Source: CAD feature listing. Evaluate the final solid. Frame: model axes, mm. Face numbers are marked on the shaded views. A direction names the side the tool comes from. Give positions to 0.01 mm unless a question says otherwise; leave off trailing zeros. Write each loop counter-clockwise with the first axis right and the second up, starting at its lowest first coordinate (ties: lowest second). Pieces come first, ordered by that corner, then holes.
```python
from build123d import *

# Parameters (mm, degrees)
SKETCH1_R                 = 7.5
EXTRUDE1_DEPTH            = 3
SKETCH2_R                 = 30
EXTRUDE2_DEPTH            = 6
SKETCH3_R                 = 18.5
CUT_EXTRUDE1_DEPTH        = 45.09081537
CUT_EXTRUDE2_DEPTH        = 45.09081537
SKETCH8_R                 = 18.75
EXTRUDE3_DEPTH            = 45.09081537
CIRPATTERN1_COUNT         = 5
SKETCH5_R                 = 3.05
CUT_EXTRUDE3_DEPTH        = 44.640169222
M3X0_5_TAPPED_HOLE1_D     = 2.5
M3X0_5_TAPPED_HOLE1_DEPTH = 7.5
M3X0_5_TAPPED_HOLE1_TIP   = 0.751075774


with BuildPart() as part:
    # Sketch1 → Extrude1 (new, symmetric)
    with BuildSketch(Plane.XY):
        Circle(SKETCH1_R)
    extrude(amount=EXTRUDE1_DEPTH, both=True)

    # Sketch2 → Extrude2 (add)
    with BuildSketch(Plane(origin=(0, 0, -3), x_dir=(-1, 0, 0), z_dir=(0, 0, -1))):
        Circle(SKETCH2_R)
    extrude(amount=EXTRUDE2_DEPTH)

    # Sketch3 → Cut-Extrude1 (cut, through all)
    with BuildSketch(Plane(origin=(0, 0, -9), x_dir=(-1, 0, 0), z_dir=(0, 0, -1))):
        with Locations((0, -38)):
            Circle(SKETCH3_R)
    cut_extrude1 = extrude(amount=-CUT_EXTRUDE1_DEPTH, mode=Mode.SUBTRACT)

    # Sketch4 → Cut-Extrude2 (cut, through all)
    with BuildSketch(Plane(origin=(0, 0, -9), x_dir=(-1, 0, 0), z_dir=(0, 0, -1))):
        with BuildLine():
            Line((6.794236298, -13.604718046), (15.549680784, -25.655553542))
            ThreePointArc((15.549680784, -25.655553542), (17.633557569, -24.270509831), (19.594765756, -22.71662728))
            Line((19.594765756, -22.71662728), (10.83932127, -10.665791785))
            ThreePointArc((10.83932127, -10.665791785), (7.347315654, -10.11271243), (6.794236298, -13.604718046))
        make_face()
    cut_extrude2 = extrude(amount=-CUT_EXTRUDE2_DEPTH, mode=Mode.SUBTRACT)

    # Sketch8 → Extrude3 (cut, through all)
    with BuildSketch(Plane(origin=(0, 0, -9), x_dir=(-1, 0, 0), z_dir=(0, 0, -1))):
        with Locations((0, -38)):
            Circle(SKETCH8_R)
    extrude3 = extrude(amount=-EXTRUDE3_DEPTH, mode=Mode.SUBTRACT)

    # CirPattern1: Cut-Extrude1, Cut-Extrude2, Extrude3 ×5 about axis
    cirpattern1_axis = Axis((0, 0, 0), (0, 0, 1))
    add([cut_extrude1.rotate(cirpattern1_axis, i * 360 / CIRPATTERN1_COUNT) for i in range(1, CIRPATTERN1_COUNT)], mode=Mode.SUBTRACT)
    add([cut_extrude2.rotate(cirpattern1_axis, i * 360 / CIRPATTERN1_COUNT) for i in range(1, CIRPATTERN1_COUNT)], mode=Mode.SUBTRACT)
    add([extrude3.rotate(cirpattern1_axis, i * 360 / CIRPATTERN1_COUNT) for i in range(1, CIRPATTERN1_COUNT)], mode=Mode.SUBTRACT)

    # Sketch5 → Cut-Extrude3 (cut, through all)
    with BuildSketch(Plane(origin=(0, 0, -9), x_dir=(-1, 0, 0), z_dir=(0, 0, -1))):
        Circle(SKETCH5_R)
    extrude(amount=-CUT_EXTRUDE3_DEPTH, mode=Mode.SUBTRACT)

    # M3x0.5 Tapped Hole1
    with Locations(Plane(origin=(0, 7.5, 0), x_dir=(-1, 0, 0), z_dir=(0, 1, 0))):
        with Locations((0, 0)):
            Hole(M3X0_5_TAPPED_HOLE1_D / 2, depth=M3X0_5_TAPPED_HOLE1_DEPTH)
            with Locations((0, 0, -(M3X0_5_TAPPED_HOLE1_DEPTH + M3X0_5_TAPPED_HOLE1_TIP / 2))):  # 118° drill point
                Cone(0, M3X0_5_TAPPED_HOLE1_D / 2, M3X0_5_TAPPED_HOLE1_TIP, mode=Mode.SUBTRACT)


solid = part.part
```
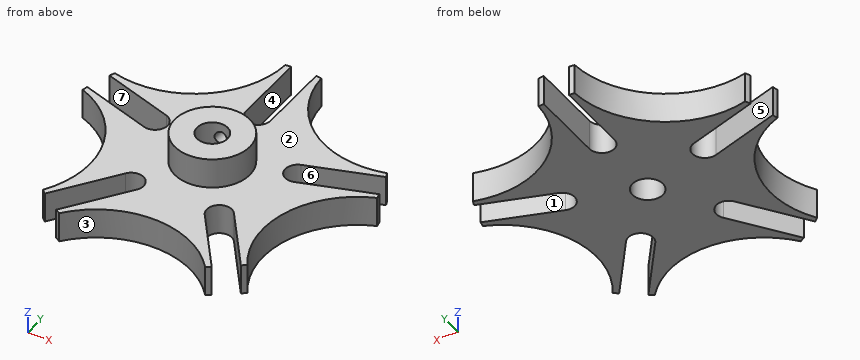
1. Mould query, pull axis Y, two halves, no side actions, for the marked faces 1, 2 and 3. Classes: +Y half, -Y half, draft (parallel to the pull), parting line (faces both ways), or undercut.
2. Line query: L1, parallel to Z at x = 0, y = 6.55; L2, parallel to X at y = 0.5, z = 2; L3, parallel to Y at x = 0, z = -2. Output: solid intervals per line, ascending.
3. Contact query for flat-ended pins moving along their axis: P1, Ø12, axis at x = 14.5, y = 11.5, coming from the +Z side; P2, Ø6, axis at x = 6, z = 1, coming from the -Y side; P3, Ø2, axis at x = 0, z = 0, coming from the -Y side; P4, Ø2, axis at x = 17, z = -0.5, coming from the -Y side. Output: stop coordinate, or through.
4. Cut plane D-D, the plane y = -16.5. Return the cut outline in (x, z), then the cut area to 3 significant figures.
5. Cut plane B-B, the plane y = 0. Return the cut outline in (x, z).
6. Access query for the marked faces 4, 5, 6 and 7. Directions: +Z, -Z, +X, -X, +Y, -Y. A direction counts if a zero-diameter tool reaches every point of the face in a straight line with its end or side. Return the directions, or none.
7. Cut plane A-A, the plane x = 0. Return the cut outline in (y, z).
Response values:
1. face 1: undercut
1. face 2: draft
1. face 3: -Y half
2. L1: z = -9 to -1.25, 1.25 to 3
2. L2: x = -7.48 to -3.01, 3.01 to 7.48
2. L3: y = -7.5 to -3.05, 3.05 to 7.5
3. P1: stops at z = -3
3. P2: stops at y = -6.87
3. P3: stops at y = -7.5
3. P4: passes through
4. outline: (-18, -9) - (-15.08, -9) - (-15.08, -3) - (-18, -3) - close; (-8.9, -9) - (8.9, -9) - (8.9, -3) - (-8.9, -3) - close; (15.08, -9) - (18, -9) - (18, -3) - (15.08, -3) - close
4. area: 142 mm2
5. outline: (-21.52, -9) - (-3.05, -9) - (-3.05, 3) - (-7.5, 3) - (-7.5, -3) - (-21.52, -3) - close; (3.05, -9) - (21.52, -9) - (21.52, -3) - (7.5, -3) - (7.5, 3) - (3.05, 3) - close
6. face 4: +Z, -Z, +Y
6. face 5: +Z, -Z
6. face 6: +Z, -Z, +X
6. face 7: +Z, -Z, -X
7. outline: (-19.25, -9) - (-3.05, -9) - (-3.05, 3) - (-7.5, 3) - (-7.5, -3) - (-19.25, -3) - close; (3.05, -9) - (12.5, -9) - (12.5, -3) - (7.5, -3) - (7.5, -1.25) - (3.05, -1.25) - close; (3.05, 1.25) - (7.5, 1.25) - (7.5, 3) - (3.05, 3) - close
